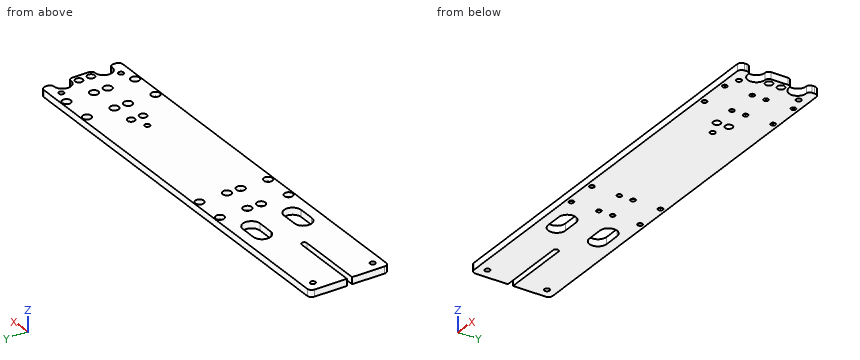
from build123d import *

# Parameters (mm, degrees)
SKETCH_R     = 2.8
SKETCH_R_2   = 4.25
SKETCH_R_3   = 3
PAD_DEPTH    = 8
SKETCH001_R  = 5
POCKET_DEPTH = 5.5


with BuildPart() as part:
    # Sketch → Pad (new body)
    with BuildSketch(Plane.XY):
        with BuildLine():
            Line((-5, 46), (-470, 46))
            ThreePointArc((-470, 46), (-473.535534, 44.535534), (-475, 41))
            Line((-475, 41), (-475, 3))
            Line((-395, 3), (-475, 3))
            ThreePointArc((-395, -3), (-392, 0), (-395, 3))
            Line((-395, -3), (-475, -3))
            Line((-475, -3), (-475, -41))
            ThreePointArc((-475, -41), (-473.535534, -44.535534), (-470, -46))
            Line((-5, -46), (-470, -46))
            ThreePointArc((-5, -46), (-1.464466, -44.535534), (0, -41))
            Line((0, -41), (0, -37.991069))
            ThreePointArc((0, -37.991069), (-1.22254, -35.112577), (-4.142857, -33.99362))
            ThreePointArc((-4.142857, -14.00638), (-14.5, -24), (-4.142857, -33.99362))
            ThreePointArc((-4.142857, -14.00638), (-1.22254, -12.887423), (0, -10.008931))
            Line((0, 10.008931), (0, -10.008931))
            ThreePointArc((0, 10.008931), (-1.22254, 12.887423), (-4.142857, 14.00638))
            ThreePointArc((-4.142857, 33.99362), (-14.5, 24), (-4.142857, 14.00638))
            ThreePointArc((-4.142857, 33.99362), (-1.22254, 35.112577), (0, 37.991069))
            Line((0, 41), (0, 37.991069))
            ThreePointArc((0, 41), (-1.464466, 44.535534), (-5, 46))
        make_face()
        with Locations((-306.75, 40)):
            Circle(SKETCH_R, mode=Mode.SUBTRACT)
        with Locations((-270.75, 40)):
            Circle(SKETCH_R, mode=Mode.SUBTRACT)
        with Locations((-270.75, 8)):
            Circle(SKETCH_R, mode=Mode.SUBTRACT)
        with Locations((-306.75, 8)):
            Circle(SKETCH_R, mode=Mode.SUBTRACT)
        with Locations((-306.75, -8)):
            Circle(SKETCH_R, mode=Mode.SUBTRACT)
        with Locations((-270.75, -8)):
            Circle(SKETCH_R, mode=Mode.SUBTRACT)
        with Locations((-306.75, -40)):
            Circle(SKETCH_R, mode=Mode.SUBTRACT)
        with Locations((-270.75, -40)):
            Circle(SKETCH_R, mode=Mode.SUBTRACT)
        with Locations((-72, -40)):
            Circle(SKETCH_R, mode=Mode.SUBTRACT)
        with Locations((-36, -40)):
            Circle(SKETCH_R, mode=Mode.SUBTRACT)
        with Locations((-36, -8)):
            Circle(SKETCH_R, mode=Mode.SUBTRACT)
        with Locations((-72, -8)):
            Circle(SKETCH_R, mode=Mode.SUBTRACT)
        with Locations((-36, 8)):
            Circle(SKETCH_R, mode=Mode.SUBTRACT)
        with Locations((-36, 40)):
            Circle(SKETCH_R, mode=Mode.SUBTRACT)
        with Locations((-72, 40)):
            Circle(SKETCH_R, mode=Mode.SUBTRACT)
        with Locations((-72, 8)):
            Circle(SKETCH_R, mode=Mode.SUBTRACT)
        with Locations((-100, 7)):
            Circle(SKETCH_R_2, mode=Mode.SUBTRACT)
        with Locations((-100, -7)):
            Circle(SKETCH_R_2, mode=Mode.SUBTRACT)
        with Locations((-8, 7)):
            Circle(SKETCH_R_2, mode=Mode.SUBTRACT)
        with Locations((-8, -7)):
            Circle(SKETCH_R_2, mode=Mode.SUBTRACT)
        with Locations((-19, 34.8)):
            Circle(SKETCH_R_3, mode=Mode.SUBTRACT)
        with Locations((-463, 34.8)):
            Circle(SKETCH_R_3, mode=Mode.SUBTRACT)
        with Locations((-463, -34.8)):
            Circle(SKETCH_R_3, mode=Mode.SUBTRACT)
        with Locations((-19, -34.8)):
            Circle(SKETCH_R_3, mode=Mode.SUBTRACT)
        with Locations((-118, 0)):
            Circle(SKETCH_R_3, mode=Mode.SUBTRACT)
        with BuildLine():
            ThreePointArc((-356.75, 34), (-366.75, 24), (-356.75, 14))
            Line((-356.75, 14), (-338.25, 14))
            ThreePointArc((-338.25, 14), (-328.25, 24), (-338.25, 34))
            Line((-356.75, 34), (-338.25, 34))
        make_face(mode=Mode.SUBTRACT)
        with BuildLine():
            ThreePointArc((-356.75, -14), (-366.75, -24), (-356.75, -34))
            Line((-356.75, -34), (-338.25, -34))
            ThreePointArc((-338.25, -34), (-328.25, -24), (-338.25, -14))
            Line((-356.75, -14), (-338.25, -14))
        make_face(mode=Mode.SUBTRACT)
    extrude(amount=-PAD_DEPTH)

    # Sketch001 → Pocket (cut)
    with BuildSketch(Plane.XY):
        with Locations((-306.75, -40)):
            Circle(SKETCH001_R)
        with Locations((-36, 8)):
            Circle(SKETCH001_R)
        with Locations((-36, 40)):
            Circle(SKETCH001_R)
        with Locations((-36, -40)):
            Circle(SKETCH001_R)
        with Locations((-270.75, -8)):
            Circle(SKETCH001_R)
        with Locations((-72, -40)):
            Circle(SKETCH001_R)
        with Locations((-306.75, 40)):
            Circle(SKETCH001_R)
        with Locations((-72, -8)):
            Circle(SKETCH001_R)
        with Locations((-270.75, 40)):
            Circle(SKETCH001_R)
        with Locations((-270.75, 8)):
            Circle(SKETCH001_R)
        with Locations((-72, 8)):
            Circle(SKETCH001_R)
        with Locations((-270.75, -40)):
            Circle(SKETCH001_R)
        with Locations((-72, 40)):
            Circle(SKETCH001_R)
        with Locations((-306.75, -8)):
            Circle(SKETCH001_R)
        with Locations((-36, -8)):
            Circle(SKETCH001_R)
        with Locations((-306.75, 8)):
            Circle(SKETCH001_R)
    extrude(amount=-POCKET_DEPTH, mode=Mode.SUBTRACT)


solid = part.part
The model under review builds one solid part; all positions refer to its coordinate system, in mm. Round coordinates to 2 decimals unless told otherwise and drop trailing zeros. Loops run counter-clockwise (first coordinate to the right, second up) from the corner with the lowest first, then second, coordinate; pieces in that order, holes last. Notation, with made-up numbers: (65.25, -18.75) - (110.25, -18.75) arc R26 ccw to (110.25, 13.25) - close; hole circle Ø9 at (-20, 35). An arc over 180 degrees is marked (long way). Use CSV: the item, a comma, the result in double quotes.
(1) Clearance check with flat-ended pins moving along their axes: P1, Ø3.5, axis at x = -306.75, y = 40, coming from the +Z side; P2, Ø1.5, axis at y = -35, z = -1, coming from the +X side; P3, Ø6, axis at x = -36, y = 40, coming from the +Z side; P4, Ø2, axis at y = 16.5, z = -6.5, coming from the +X side. State where each tip first meets the part, or that it passes through.
Working result:
P1,"passes through"
P2,"stops at x = -0.69"
P3,"stops at z = -5.5"
P4,"stops at x = -9.77"
(2) Take a section at C-C, the plane x = -417.5. Give the boundary of the cut face in (y, z).
Working result:
outline,"(-46, -8) - (-3, -8) - (-3, 0) - (-46, 0) - close; (3, -8) - (46, -8) - (46, 0) - (3, 0) - close"
(3) Take a section at A-A, the plane y = 24. Give the boundary of the cut face in (x, z).
Working result:
outline,"(-475, -8) - (-366.75, -8) - (-366.75, 0) - (-475, 0) - close; (-328.25, -8) - (-14.5, -8) - (-14.5, 0) - (-328.25, 0) - close"
(4) For line 1 (Y direction, x = -306.75, z = -6.3); line 2 (Y direction, x = -72, z = -1.5); line 3 (Y direction, x = -445, z = -0.25), list the stretches that pass through material, from the lowest coordinate up.
Working result:
line 1,"y = -46 to -42.8, -37.2 to -10.8, -5.2 to 5.2, 10.8 to 37.2, 42.8 to 46"
line 2,"y = -46 to -45, -35 to -13, -3 to 3, 13 to 35, 45 to 46"
line 3,"y = -46 to -3, 3 to 46"
(5) Take a section at D-D, the plane z = -2.75. State how many separate pieces and enclosed holes the cut face has, plus the area to 3 significant figures.
Working result:
separate pieces,"1"
enclosed holes,"27"
area,"39,700 mm^2"
(6) Take a section at B-B, the plane x = -100. Give the boundary of the cut face in (y, z).
Working result:
outline,"(-46, -8) - (-11.25, -8) - (-11.25, 0) - (-46, 0) - close; (-2.75, -8) - (2.75, -8) - (2.75, 0) - (-2.75, 0) - close; (11.25, -8) - (46, -8) - (46, 0) - (11.25, 0) - close"
